Verification items for this drawing (mm, ordinates from the low corner). A direction names the side the tool comes from. Coordinates: 2 decimals unless noted, no trailing zeros. Write each loop counter-clockwise with the first axis right and the second up, starting at its lowest first coordinate (ties: lowest second). Pieces come first, ordered by that corner, then holes. Notation, with made-up numbers: (10.25, 56) -> (65.25, 56) arc R12 cw to (65.25, 62) -> close; hole circle Ø6 at (82, -12). An arc over 180 degrees is marked (long way). Put each result on its own line as item: value. Start each with the question number.
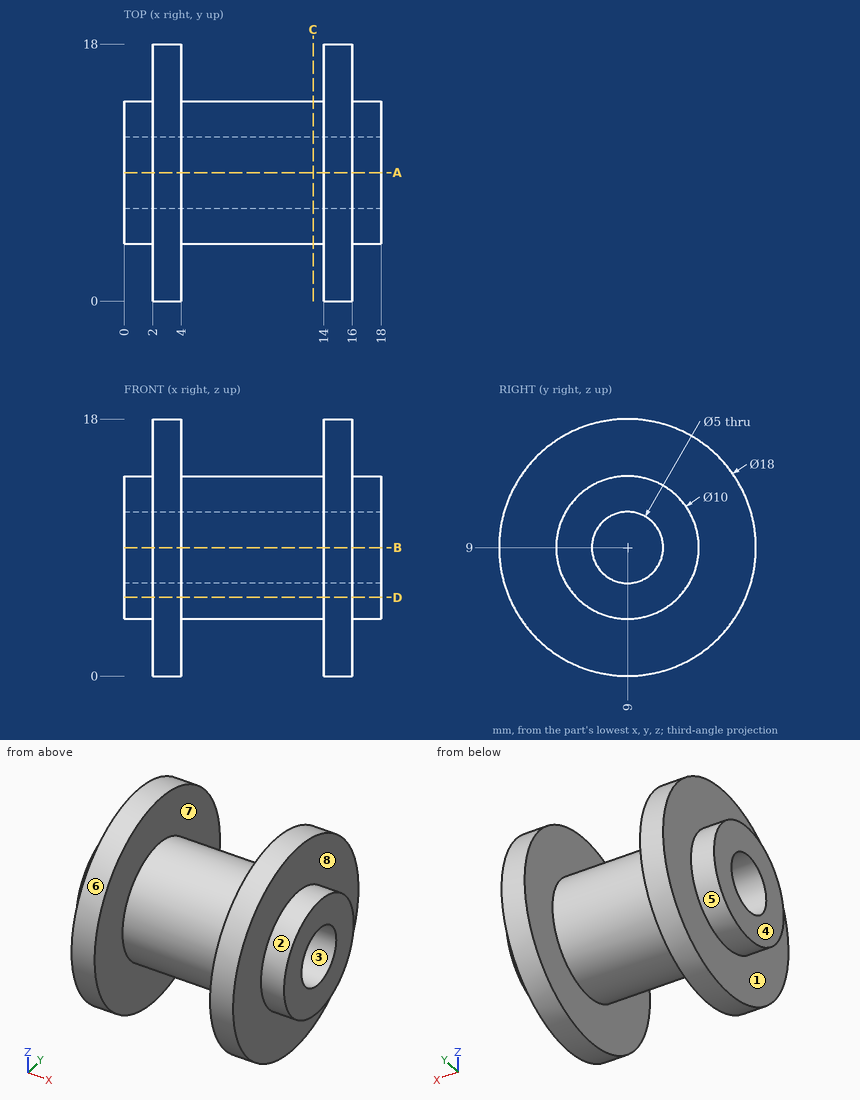
Item 1: Section check C-C, the plane x = 13.25. Enter the section's corners in (y, z), and give its area (3 significant figures).
Item 2: Scan lines: line 1 along Y through (x, z) = (5.5, 9); line 2 along X through (y, z) = (1, 12.25); line 3 along Z through (x, y) = (11, 8). Record each from-to range of solid material in increasing order. Write a range as [from, to].
Item 3: Section check A-A, the plane y = 9. Enter the section's corners in (x, z).
Item 4: Mould release check, pull along Z, two halves, no side actions. Record for the marked faces 1, 2 and 3: released by +Z, released by -Z, zero draft, split by the parting line, or undercut.
Item 5: Go/stop test with flat-tipped pins: P1, Ø1.5, axis at x = 15, z = 10, coming from the -Y side; P2, Ø5, axis at x = 8, y = 9.5, coming from the -Z side; P3, Ø6, axis at y = 3, z = 13.5, coming from the +X side; P4, Ø1, axis at x = 7, z = 12.5, coming from the -Y side. Record where each tip stops, or that it passes through.
Item 6: Access from +Z, -Z, +X, -X, +Y, -Y to the whole of each face (thin tool, end or side, straight path). Record for the marked faces 4, 5, 6, 7 and 8.
Item 7: Section check D-D, the plane z = 5.5. Enter the section's corners in (x, y).
From the geometry:
1. outline: circle Ø10 at (9, 9); hole circle Ø5 at (9, 9)
1. area: 58.9 mm²
2. line 1: [4, 6.5], [11.5, 14]
2. line 2: [2, 4], [14, 16]
2. line 3: [4.1, 6.71], [11.29, 13.9]
3. outline: (0, 4) -> (2, 4) -> (2, 0) -> (4, 0) -> (4, 4) -> (14, 4) -> (14, 0) -> (16, 0) -> (16, 4) -> (18, 4) -> (18, 6.5) -> (0, 6.5) -> close; (0, 11.5) -> (18, 11.5) -> (18, 14) -> (16, 14) -> (16, 18) -> (14, 18) -> (14, 14) -> (4, 14) -> (4, 18) -> (2, 18) -> (2, 14) -> (0, 14) -> close
4. face 1: zero draft
4. face 2: split by the parting line
4. face 3: undercut
5. P1: y = 0
5. P2: z = 4
5. P3: x = 18
5. P4: y = 5
6. face 4: +Z, -Z, -X, +Y, -Y
6. face 5: -X
6. face 6: +X, -X
6. face 7: none
6. face 8: +X
7. outline: (0, 5.43) -> (2, 5.43) -> (2, 0.71) -> (4, 0.71) -> (4, 5.43) -> (14, 5.43) -> (14, 0.71) -> (16, 0.71) -> (16, 5.43) -> (18, 5.43) -> (18, 12.57) -> (16, 12.57) -> (16, 17.29) -> (14, 17.29) -> (14, 12.57) -> (4, 12.57) -> (4, 17.29) -> (2, 17.29) -> (2, 12.57) -> (0, 12.57) -> close
